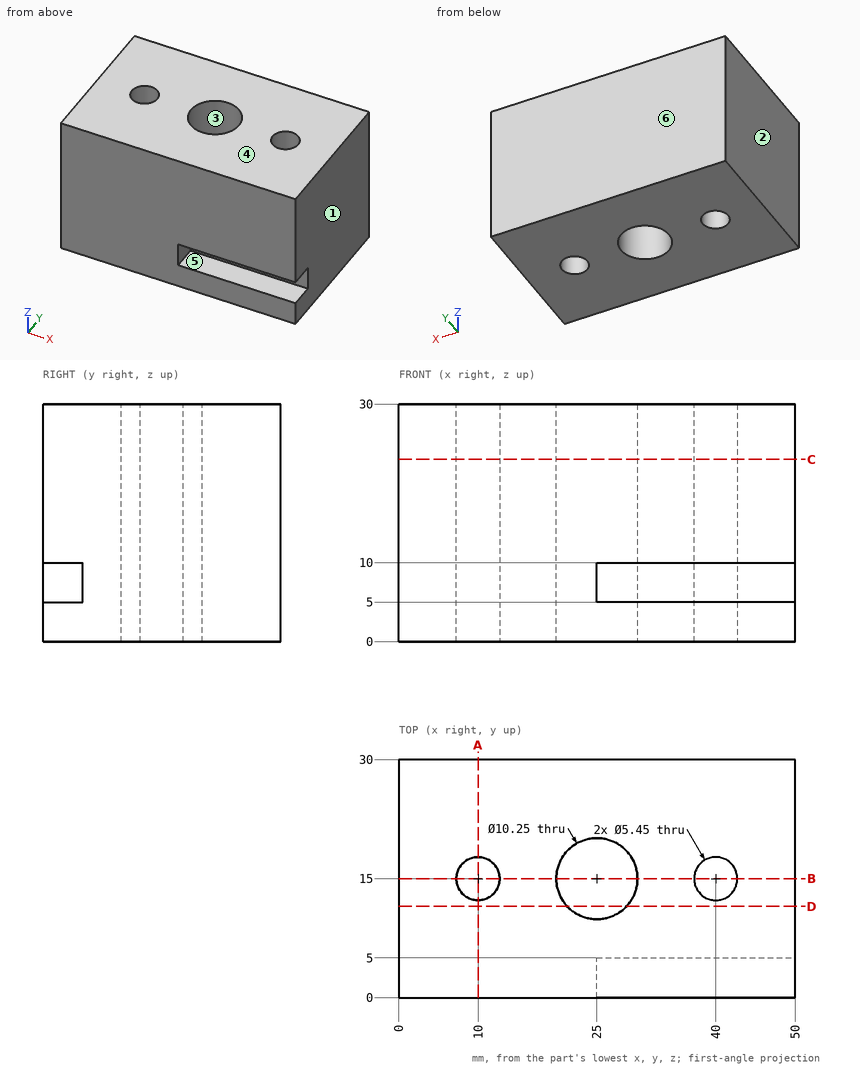
Input: dimensioned drawing with shaded views. Units: mm. Origin: part minimum x, y, z. A direction names the side the tool comes from. Round coordinates to 2 decimals unless told otherwise and drop trailing zeros. Order: outer loops, then holes, each group sorted by start corner. A loop starts at its lowest first (then second) coordinate and runs counter-clockwise, first axis right, second up.
1. Material intervals for line 1 (Y direction, x = 25, z = 19.5) (3 decimals); line 2 (Y direction, x = 40, z = 20.25) (3 decimals); line 3 (Z direction, x = 31, y = 4.5), sorted ascending.
The answers:
line 1: y = 0 to 9.875, 20.125 to 30
line 2: y = 0 to 12.275, 17.725 to 30
line 3: z = 0 to 5, 10 to 30
2. Cut plane A-A, the plane x = 10. Output: boundary loops of the cut face in (y, z) (3 decimals), then the cut area to 4 significant figures.
The answers:
outline: (0, 0) - (12.275, 0) - (12.275, 30) - (0, 30) - close; (17.725, 0) - (30, 0) - (30, 30) - (17.725, 30) - close
area: 736.5 mm2
3. Cut plane D-D, the plane y = 11.5. Output: boundary loops of the cut face in (x, z), then the cut area to 3 significant figures.
The answers:
outline: (0, 0) - (21.26, 0) - (21.26, 30) - (0, 30) - close; (28.74, 0) - (50, 0) - (50, 30) - (28.74, 30) - close
area: 1,280 mm2
4. Set-up query: the marked faces 5 and 6. Return all of +Z, -Z, +X, -X, +Y, -Y with unobstructed straight access to the full face (end or side cutting, diameter ignored); none if empty.
The answers:
face 5: +X, -Y
face 6: +Z, -Z, +X, -X, +Y
5. Cut plane B-B, the plane y = 15. Output: boundary loops of the cut face in (x, z) (3 decimals).
The answers:
outline: (0, 0) - (7.275, 0) - (7.275, 30) - (0, 30) - close; (12.725, 0) - (19.875, 0) - (19.875, 30) - (12.725, 30) - close; (30.125, 0) - (37.275, 0) - (37.275, 30) - (30.125, 30) - close; (42.725, 0) - (50, 0) - (50, 30) - (42.725, 30) - close
6. Pin query (flat end, axial travel): P1, Ø9, axis at x = 25, y = 15, coming from the -Z side; P2, Ø2.5, axis at y = 2.5, z = 8, coming from the +X side. Return the tip coordinate at first contact, or that it passes through.
The answers:
P1: passes through
P2: stops at x = 25
7. Mould query, pull axis X, two halves, no side actions, for the marked faces 1, 2, 3 and 4. Classes: released by +X, released by -X, zero draft, split by the parting line, or undercut.
The answers:
face 1: released by +X
face 2: released by -X
face 3: undercut
face 4: zero draft
8. Cut plane C-C, the plane z = 23. Output: boundary loops of the cut face in (x, y) (3 decimals), then the cut area to 3 significant figures.
The answers:
outline: (0, 0) - (50, 0) - (50, 30) - (0, 30) - close; hole circle Ø5.45 at (10, 15); hole circle Ø10.25 at (25, 15); hole circle Ø5.45 at (40, 15)
area: 1,370 mm2
